Input: part model. Units: mm. Frame: model coordinates. Face numbers are marked on the shaded views. A direction names the side the tool comes from. Round coordinates to 2 decimals unless told otherwise and drop trailing zeros. Loops run counter-clockwise (first coordinate to the right, second up) from the corner with the lowest first, then second, coordinate; pieces in that order, holes last.
(1) Cut plane B-B, the plane y = 0. Give the number of separate pieces and of enclosed holes in the cut face, and give its area (3 significant figures).
(2) First-contact query: pin 1 Ø5.5 at (x, z) = (61, 12.5) entering from -Y; pin 2 Ø12 at (y, z) = (-9, 11) entering from -X; pin 3 Ø4 at (x, y) = (-49.3, 13.3) entering from +Z; pin 4 Ø10.5 at (x, y) = (62.5, -3) entering from +Z. Flat tips, straight axial feed; report the tip coordinate or a pass-through.
(3) Cut plane D-D, the plane x = 62. Output: boundary loops of the cut face in (y, z).
(4) Cut plane A-A, the plane x = 11.5. Output: boundary loops of the cut face in (y, z).
(5) Line query: line 1 (X direction, y = -5, z = 1.25); line 2 (X direction, y = 0, z = -2.7); line 3 (Y direction, x = -50.5, z = -1). Output: solid intervals per line, ascending.
(6) Access query for the marked faces 1 and 2. Directions: +Z, -Z, +X, -X, +Y, -Y. A direction counts if a zero-diameter tool reaches every point of the face in a straight line with its end or side. Return the directions, or none.
(7) Cut plane C-C, the plane z = 6.5. Output: boundary loops of the cut face in (x, y), and give its area (3 significant figures).
(8) Draft query along Y for the marked faces 3, 4 and 5. Return one class per face: released by +Y, released by -Y, zero draft, split by the parting line, or undercut.
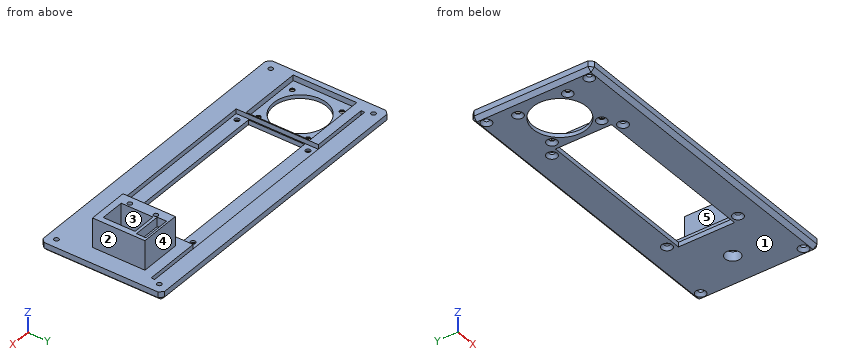
Autodesk Inventor part; units mm, degrees
ref_plane "YZ Plane" through (0, 0, 0) normal (1, 0, 0) x (0, 1, 0)
ref_plane "XZ Plane" through (0, 0, 0) normal (0, 1, 0) x (-1, 0, 0)
ref_plane "XY Plane" through (0, 0, 0) normal (0, 0, 1) x (1, 0, 0)
sketch "Esquisse1" plane through (0, 0, 0) normal (0, 0, 1) x (1, 0, 0)
  line L0 (-82.5, -32.5) -> (82.5, -32.5)
  line L1 (82.5, -32.5) -> (82.5, 32.5)
  line L2 (82.5, 32.5) -> (-82.5, 32.5)
  line L3 (-82.5, 32.5) -> (-82.5, -32.5)
  line L4 (-115.5, 0) -> (115.5, 0)
  line L5 (0, -45.5) -> (0, 45.5)
  line L6 (-44.5, 15) -> (44.5, 15)
  line L7 (44.5, 15) -> (44.5, -15)
  line L8 (44.5, -15) -> (-44.5, -15)
  line L9 (-44.5, -15) -> (-44.5, 15)
  line L10 (-44.6, 22) -> (44.6, 22)
  line L11 (44.6, 22) -> (44.6, -22)
  line L12 (44.6, -22) -> (-44.6, -22)
  line L13 (-44.6, -22) -> (-44.6, 22)
  circle A0 centre (-41.6, 19) radius 1.3
  circle A1 centre (41.6, 19) radius 1.3
  circle A2 centre (-41.6, -19) radius 1.3
  circle A3 centre (41.6, -19) radius 1.3
  line L14 (-45.6, -17) -> (-79.6, -17)
  line L15 (-79.6, -17) -> (-79.6, 17)
  line L16 (-79.6, 17) -> (-45.6, 17)
  line L17 (-45.6, 17) -> (-45.6, -17)
  circle A4 centre (-49.3, -13.3) radius 1.25
  circle A5 centre (-49.3, 13.3) radius 1.25
  circle A6 centre (-73.9, -13.3) radius 1.25
  circle A7 centre (-73.9, 13.3) radius 1.25
  circle A8 centre (-61.6, 0) radius 14.25
  circle A9 centre (-77.5, -27.5) radius 1.25
  circle A10 centre (77.5, -27.5) radius 1.25
  circle A11 centre (-77.5, 27.5) radius 1.25
  circle A12 centre (77.5, 27.5) radius 1.25
  circle A13 centre (63.55, 0) radius 4
  line L18 (-76, 23.9) -> (76, 23.9)
  line L19 (76, 23.9) -> (76, 22)
  line L20 (76, 22) -> (-76, 22)
  line L21 (-76, 22) -> (-76, 23.9)
  line L22 (82.5, 32.5) -> (-82.5, 32.5)
  line L23 (-82.5, 32.5) -> (-82.5, 30.5)
  line L24 (-82.5, 30.5) -> (82.5, 30.5)
  line L25 (82.5, 30.5) -> (82.5, 32.5)
  line L26 (-44.6, -22) -> (-45.1, -22)
  line L27 (-45.1, -22) -> (-45.1, 22)
  line L28 (-45.1, 22) -> (-44.6, 22)
  line L29 (-44.6, 22) -> (-44.6, -22)
  line L30 (44.6, -22) -> (45.6, -22)
  line L31 (45.6, -22) -> (45.6, 22)
  line L32 (45.6, 22) -> (44.6, 22)
  line L33 (44.6, 22) -> (44.6, -22)
  point P0 (0, 0)
  point P1 (82.5, 30.5)
  point P2 (-44.6, 0)
  point P3 (-45.1, 0)
  dimension "d0" = 165
  dimension "d1" = 65
  dimension "d2" = 30
  dimension "d3" = 89
  dimension "d4" = 89.2
  dimension "d6" = 2.6
  dimension "d31" = 34
  dimension "d32" = 34
  dimension "d33" = 1
  dimension "d34" = 2.5
  dimension "d35" = 3.7
  dimension "d36" = 3.7
  dimension "d39" = 24.6
  dimension "d44" = 28.5
  dimension "d45" = 16
  dimension "d53" = 2.5
  dimension "d54" = 5
  dimension "d55" = 5
  dimension "d58" = 155
  dimension "d68" = 8
  dimension "d116" = 44.6
  dimension "d119" = 63.55
  dimension "d122" = 22
  dimension "d124" = 44.6
  dimension "d125" = 22
  dimension "d127" = 152
  dimension "d128" = 1.9
  dimension "d131" = 2
  dimension "d134" = 41.6
  dimension "d135" = 19
  dimension "d136" = 82.5
  dimension "d137" = 30.5
  dimension "d138" = 44.6
  dimension "d139" = 22
  dimension "d140" = 41.6
  dimension "d141" = 44.6
  dimension "d142" = 22
  dimension "d143" = 0.5
  dimension "d144" = 1
extrude "Extrusion1" add sketch "Esquisse1" against normal blind 5 contours L3 L4 L15 L14 L17 L27 L26 L12 L5 L0 | L5 L12 L30 L31 L4 A13 L1 L0 | L3 L24 L5 L18 L21 L20 L27 L4 L17 L16 L15 | L12 L13 L4 L9 L8 L5 | L5 L8 L7 L4 L11 L12 | L3 L2 L5 L24 | L15 L16 L17 L4 A8 | L4 A8 L17 L14 L15 | L4 A13 L31 L20 L19 L18 L5 L24 L1 | L11 L4 L31 L30 | L26 L27 L4 L13 | L5 L2 L1 L24 | A8 L4 | L4 A8 | A13 L4 | L4 A13 | L11 L20 L31 L4 | L4 L7 L6 L5 L10 L11 | L13 L10 L5 L6 L9 L4 | L4 L27 L20 L13 | L18 L19 L20 L10 L5 | L5 L10 L20 L21 L18 | A4 | A5 | A6 | A7 | A9 | A10 | A11 | A12
extrude "Extrusion2" cut sketch "Esquisse1" against normal blind 2.5 contours L12 L13 L4 L9 L8 L5 | L5 L8 L7 L4 L11 L12 | L8 L9 L4 L5 | L5 L4 L7 L8 | L11 L4 L31 L30 | L26 L27 L4 L13 | L5 L6 L7 L4 | L4 L9 L6 L5 | L11 L20 L31 L4 | L4 L7 L6 L5 L10 L11 | L13 L10 L5 L6 L9 L4 | L4 L27 L20 L13
chamfer "Chanfrein1" distance 1.5 angle 45 4 edges at (40.3, 19, -5) (-42.9, 19, -5) (40.3, -19, -5) (-42.9, -19, -5)
extrude "Extrusion3" cut sketch "Esquisse1" against normal through all contours A8 L4 | L4 A8 | A4 | A5 | A6 | A7
extrude "Extrusion4" cut sketch "Esquisse1" against normal blind 3 contours L15 L16 L17 L4 A8 | L4 A8 L17 L14 L15
chamfer "Chanfrein2" distance 1.5 angle 45 4 edges at (-75.15, 13.3, -5) (-50.55, -13.3, -5) (-75.15, -13.3, -5) (-50.55, 13.3, -5)
extrude "Extrusion5" cut sketch "Esquisse1" against normal through all contours A9 | A10 | A11 | A12
chamfer "Chanfrein3" distance 1.5 angle 45 4 edges at (-78.75, -27.5, -5) (-78.75, 27.5, -5) (76.25, -27.5, -5) (76.25, 27.5, -5)
extrude "Extrusion6" cut sketch "Esquisse1" against normal through all contours A13 L4 | L4 A13
sketch "Esquisse3" plane through (0, 0, 0) normal (0, 0, 1) x (1, 0, 0)
  line L0 (70.05, -8) -> (57.05, -8)
  line L1 (57.05, -8) -> (57.05, 9)
  line L2 (57.05, 9) -> (70.05, 9)
  line L3 (70.05, 9) -> (70.05, -8)
  circle A0 centre (63.55, 0) radius 4
  line L4 (-115.5, 0) -> (115.5, 0)
  line L5 (73.05, -11.5) -> (51.05, -11.5)
  line L6 (51.05, -11.5) -> (51.05, 16.5)
  line L7 (51.05, 16.5) -> (73.05, 16.5)
  line L8 (73.05, 16.5) -> (73.05, -11.5)
  line L9 (63.55, -11.5) -> (63.55, 16.9619)
  circle A1 centre (55.05, -4.85) radius 1.2
  circle A2 centre (55.05, 9.07) radius 1.2
  point P0 (0, 0)
  dimension "d77" = 13
  dimension "d78" = 17
  dimension "d79" = 6.5
  dimension "d80" = 11.5
  dimension "d83" = 22
  dimension "d84" = 28
  dimension "d86" = 8
  dimension "d97" = 6
  dimension "d98" = 2.4
  dimension "d99" = 9.5
  dimension "d100" = 16.9619
  dimension "d101" = 9.07
  dimension "d102" = 4.85
  dimension "d103" = 18
  dimension "d104" = 18
extrude "Extrusion7" add sketch "Esquisse3" along normal blind 15.686 contours L3 L4 L8 L5 L9 L0 | L9 L5 L6 L4 L1 L0 | L3 L2 L9 L7 L8 L4 | L4 L6 L7 L9 L2 L1
sketch "Esquisse4" plane through (0, 0, 15.686) normal (0, 0, 1) x (1, 0, 0)
  line L0 (71.05, 15.5) -> (56.05, 15.5)
  line L1 (56.05, 15.5) -> (56.05, 10.5)
  line L2 (56.05, 10.5) -> (71.05, 10.5)
  line L3 (71.05, 10.5) -> (71.05, 15.5)
  line L4 (73.05, -11.5) -> (73.05, 16.5)
  line L5 (73.05, 16.5) -> (51.05, 16.5)
  line L6 (51.05, 16.5) -> (51.05, -11.5)
  point P0 (0, 0)
  dimension "d106" = 2
  dimension "d107" = 1
  dimension "d108" = 5
  dimension "d109" = 5
extrude "Extrusion8" cut sketch "Esquisse4" against normal blind 5
extrude "Extrusion10" cut sketch "Esquisse1" against normal blind 2.5 contours L18 L19 L20 L10 L5 | L5 L10 L20 L21 L18
chamfer "Chanfrein4" distance 2 angle 45 8 edges at (0, -32.5, -5) (82.5, 0, -5) (0, 32.5, -5) (-82.5, 0, -5) (82.5, -32.5, -2.5) (82.5, 32.5, -2.5) (-82.5, 32.5, -2.5) (-82.5, -32.5, -2.5)
properties part number "face_frontale" material "PVC, non plastifié"
Reported:
1. separate pieces: 4
1. enclosed holes: 0
1. area: 314 mm2
2. pin 1: stops at y = -11.5
2. pin 2: stops at x = 51.05
2. pin 3: stops at z = -3
2. pin 4: stops at z = 15.69
3. outline: (-32.5, -3) - (-30.5, -5) - (-3.69, -5) - (-3.69, 0) - (-8, 0) - (-8, 15.69) - (-11.5, 15.69) - (-11.5, 0) - (-32.5, 0) - close; (3.69, -5) - (30.5, -5) - (32.5, -3) - (32.5, 0) - (23.9, 0) - (23.9, -2.5) - (22, -2.5) - (22, 0) - (16.5, 0) - (16.5, 15.69) - (15.5, 15.69) - (15.5, 10.69) - (10.5, 10.69) - (10.5, 15.69) - (9, 15.69) - (9, 0) - (3.69, 0) - close
4. outline: (-32.5, -3) - (-30.5, -5) - (-15, -5) - (-15, -2.5) - (-22, -2.5) - (-22, 0) - (-32.5, 0) - close; (15, -5) - (30.5, -5) - (32.5, -3) - (32.5, 0) - (23.9, 0) - (23.9, -2.5) - (15, -2.5) - close
5. line 1: x = 51.05 to 53.86, 56.24 to 57.05, 70.05 to 73.05
5. line 2: x = -82.5 to -79.6, -45.6 to -44.5, 44.5 to 59.55, 67.55 to 82.5
5. line 3: y = -32.5 to -17, 17 to 22, 23.9 to 32.5
6. face 1: -Z, +X, -X, +Y, -Y
6. face 2: +Z, +X, +Y, -Y
7. outline: (51.05, -11.5) - (73.05, -11.5) - (73.05, 16.5) - (51.05, 16.5) - close; hole circle Ø2.4 at (55.05, -4.85); hole circle Ø2.4 at (55.05, 9.07); hole (57.05, -8) - (70.05, -8) - (70.05, 9) - (57.05, 9) - close
7. area: 386 mm2
8. face 3: undercut
8. face 4: released by +Y
8. face 5: zero draft
